Read the model definition and answer for the solid it produces. Units are mm, in the model's axes. A direction names the side the tool comes from. Round coordinates to 2 decimals unless told otherwise and drop trailing zeros. Order: outer loops, then holes, each group sorted by start corner. A loop starts at its lowest first (then second) coordinate and runs counter-clockwise, first axis right, second up. Notation, with made-up numbers: (16, -33.5) -> (52, -33.5) arc R33 cw to (52, 5.5) -> close; hole circle Ø1 at (-17.75, 2). An arc over 180 degrees is marked (long way). Answer as a JSON object with one key per item and string values. Group by question number.
Item 1: Section A-A, the plane x = 0 is taken. Write down the section's boundary in (y, z).
Item 2: Section B-B, the plane z = 0 is taken. Write down the section's boundary in (x, y).
Item 3: For faces 1 (the cylindrical face through (-2.44, 2.46, 0.54)), 2 (the flat face through (0, 0, 0)), 3 (the flat face through (-2, 95, -2)), determine the directions among +Z, -Z, +X, -X, +Y, -Y from which every point of the face is accessible in a straight line to the end or side of a thin tool.
Item 4: Consider probe 1 along Y at (x, z) = (-1.4, -2.5); probe 2 along Z at (x, y) = (-1.4, 11); probe 3 along Z at (x, y) = (-2.45, 80.5). Determine where each line is inside the solid, lowest interval first. Write a range as from..to.
Item 5: Section C-C, the plane y = 55 is taken. Write down the section's boundary in (x, z).
from build123d import *

# Parameters (mm, degrees)
SKETCH1_R           = 3
BOSS_EXTRUDE1_DEPTH = 100
SKETCH2_R           = 3.804683346
SKETCH2_R_2         = 2.5
CUT_EXTRUDE1_DEPTH  = 5
CUT_EXTRUDE2_START  = -5
SKETCH3_R           = 4.634260774
SKETCH3_R_2         = 2.5
CUT_EXTRUDE2_DEPTH  = 5


with BuildPart() as part:
    # Sketch1 → Boss-Extrude1 (new body)
    with BuildSketch(Plane(origin=(0, 0, 0), x_dir=(1, 0, 0), z_dir=(0, 1, 0))):
        with Locations(Location((0, 0, 0), (0, 0, 270))):
            Circle(SKETCH1_R)
    extrude(amount=BOSS_EXTRUDE1_DEPTH)

    # Sketch2 → Cut-Extrude1 (cut)
    with BuildSketch(Plane.XZ):
        Circle(SKETCH2_R)
        with Locations(Location((0, 0, 0), (0, 0, 270))):
            Circle(SKETCH2_R_2, mode=Mode.SUBTRACT)
    extrude(amount=-CUT_EXTRUDE1_DEPTH, mode=Mode.SUBTRACT)

    # Sketch3 → Cut-Extrude2 (cut)
    with BuildSketch(Plane(origin=(0, 100, 0), x_dir=(1, 0, 0), z_dir=(0, 1, 0)).offset(CUT_EXTRUDE2_START)):
        Circle(SKETCH3_R)
        with Locations(Location((0, 0, 0), (0, 0, 90))):
            Circle(SKETCH3_R_2, mode=Mode.SUBTRACT)
    extrude(amount=CUT_EXTRUDE2_DEPTH, mode=Mode.SUBTRACT)


solid = part.part
Values found:
{
 "1": {"outline": "(0, -2.5) -> (5, -2.5) -> (5, -3) -> (95, -3) -> (95, -2.5) -> (100, -2.5) -> (100, 2.5) -> (95, 2.5) -> (95, 3) -> (5, 3) -> (5, 2.5) -> (0, 2.5) -> close"},
 "2": {"outline": "(-3, 5) -> (-2.5, 5) -> (-2.5, 0) -> (2.5, 0) -> (2.5, 5) -> (3, 5) -> (3, 95) -> (2.5, 95) -> (2.5, 100) -> (-2.5, 100) -> (-2.5, 95) -> (-3, 95) -> close"},
 "3": {"face 1": "-Y", "face 2": "+Z, -Z, +X, -X, -Y", "face 3": "+Y"},
 "4": {"probe 1": "5..95", "probe 2": "-2.65..2.65", "probe 3": "-1.73..1.73"},
 "5": {"outline": "circle Ø6 at (0, 0)"}
}
